Could you check a few things on this model? Use its own coordinates, in mm. A direction names the side the tool comes from. Round coordinates to 2 decimals unless told otherwise and drop trailing zeros. Write each question's results on one line, items separated by ' | '. Start each with the question number.
(1) On a 3-axis mill with a long thin cutter (end or side, diameter ignored), from which of +Z, -Z, +X, -X, +Y, -Y can I reach the whole of each face in a straight line? I mean faces 1 (the flat face through (-55, -12, 16)), 2 (the flat face through (-51.37, -5.92, 31.8)). Say none if no direction works.
(2) Thinking about a two-plate mould opening in X: for faces 3 (the flat face through (-134.018, -6, 16)), 4 (the flat face through (-55, 0, 16)), 5 (the cylindrical face through (-1.432, -5.916, -31.474)), which applies, +X half, -X half, draft (parallel to the pull), parting line (faces both ways), or undercut?
(3) Imagine slicing it at A-A on x = 2. State how many separate pieces and enclosed holes the cut face has, then the cut area to 3 significant figures.
(4) Please list where these lines run through material, in increasing order: line 1 (Z direction, x = 0, y = -3.25); line 2 (Z direction, x = -45, y = -3.5); line 3 (X direction, y = -1.5, z = -32.5). Write a range as [from, to].
```python
from build123d import *

# Parameters (mm, degrees)
F0_R     = 11
F1_DEPTH = 12


with BuildPart() as f1:
    # F0 (on Front) → F1 (new body)
    with BuildSketch(Plane.XZ):
        with BuildLine():
            Line((25.981579, 78.608206), (-15.442509, 102.743387))
            Line((-15.442509, 102.743387), (-134.018421, 102.743387))
            Line((-134.018421, 102.743387), (-134.018421, -74.145091))
            Line((-134.018421, -74.145091), (25.981579, -74.145091))
            Line((25.981579, -74.145091), (25.981579, 30.882375))
            add(Edge.make_bspline(
                [(-48.616274, 30.909721), (-26.945135, 23.237184), (0, 20.642917), (25.981579, 30.882375)],
                knots=[0, 0, 0, 0, 74.597858, 74.597858, 74.597858, 74.597858], degree=3))
            Line((-48.616274, 30.909721), (-54.192658, 32.713946))
            ThreePointArc((-54.192658, 32.713946), (-55.161698, 33.145772), (-56.017817, 33.772328))
            ThreePointArc((-56.017817, 33.772328), (-58.570506, 46.590881), (-47.069505, 52.800428))
            add(Edge.make_bspline(
                [(-47.069505, 52.800428), (-26.67203, 45.323465), (0.517313, 43.181155), (25.981579, 52.882375)],
                knots=[1.854694, 1.854694, 1.854694, 1.854694, 74.59953, 74.59953, 74.59953, 74.59953], degree=3))
            Line((25.981579, 52.882375), (25.981579, 78.608206))
        make_face()
        with Locations((0, -42.380005)):
            Circle(F0_R, mode=Mode.SUBTRACT)
    extrude(amount=F1_DEPTH)


solid = f1.part
```
Response:
1) face 1: +Z, -Z, +X, -X, -Y | face 2: +X, +Y, -Y
2) face 3: -X half | face 4: draft | face 5: undercut
3) separate pieces: 3 | enclosed holes: 0 | area: 1,470 mm²
4) line 1: [-74.15, -53.38], [-31.38, 24.64], [46.86, 93.75] | line 2: [-74.15, 29.69], [52.07, 102.74] | line 3: [-134.02, -4.84], [4.84, 25.98]
